from build123d import *

# Parameters (mm, degrees)
SKETCH_1_R          = 0.7
EXTRUDE_1_DEPTH     = 1
CUT_EXTRUDE_1_DEPTH = 2


with BuildPart() as part:
    # Эскиз1 → Вытянуть1 (new body)
    with BuildSketch(Plane(origin=(0, 0, 0), x_dir=(0, 0, -1), z_dir=(1, 0, 0))):
        with BuildLine():
            Line((0, 0), (70, 0))
            ThreePointArc((70, 0), (72, -2), (70, -4))
            Line((70, -4), (0, -4))
            ThreePointArc((0, -4), (-2, -2), (0, 0))
        make_face()
        with Locations((0, -2)):
            Circle(SKETCH_1_R, mode=Mode.SUBTRACT)
        with Locations((70, -2)):
            Circle(SKETCH_1_R, mode=Mode.SUBTRACT)
    extrude(amount=EXTRUDE_1_DEPTH)

    # Эскиз2 → Вырез-Вытянуть1 (cut, through all)
    with BuildSketch(Plane(origin=(1, 0, 0), x_dir=(0, 0, -1), z_dir=(1, 0, 0))):
        with BuildLine():
            Line((185.588178167, -105.966859724), (69.968626967, -4))
            ThreePointArc((69.968626967, -4), (67.624087686, -2.723985874), (64.958110934, -2.591153482))
            Line((64.958110934, -2.591153482), (56.968145289, -4))
            Line((56.968145289, -4), (-94.849228607, -30.769499158))
            Line((-94.849228607, -30.769499158), (-174.701887648, -328.568151357))
            Line((-174.701887648, -328.568151357), (105.735519126, -403.765511923))
            Line((105.735519126, -403.765511923), (185.588178167, -105.966859724))
        make_face()
    extrude(amount=-CUT_EXTRUDE_1_DEPTH, mode=Mode.SUBTRACT)


solid = part.part
Model file for the job. Use its own axes, mm. Coordinates: 2 decimals unless noted, no trailing zeros. Write each loop counter-clockwise with the first axis right and the second up, starting at its lowest first coordinate (ties: lowest second). Pieces come first, ordered by that corner, then holes. Notation, with made-up numbers: (60, -33.75) -> (111, -33.75) arc R25 ccw to (111, -14.75) -> close; hole circle Ø8 at (-36.75, 55). An arc over 180 degrees is marked (long way). One line per item, written item: value. Start each with the question number.
1) Slice it at A-A on x = 0.7. Count the separate pieces of the cut face and the enclosed holes in it, then the cut area to 3 significant figures.
2) Slice it at B-B on z = -61. Write the cut outline in (x, y), then the cut area to 3 significant figures.
3) Probe probe 1 along Y at (x, z) = (0.6, -70); probe 2 along Y at (x, z) = (0.5, -57); probe 3 along Y at (x, z) = (0.7, -68.5). List the from-to ranges inside material, lowest first.
4) Flat gauge pins, fed straight in: pin 1 Ø2 at (y, z) = (-2, 0) entering from +X; pin 2 Ø1.1 at (y, z) = (-2, -70) entering from +X. Where does each tip first touch, or does it go through?
5) Pull direction Z, two halves, no side cores. Call faces 1 (the face through (0.5, -2, -69.3)), 2 (the face through (0, -2, -36)), 3 (the face through (0.5, -2, -72)), 4 (the face through (0.507, -3.286, -61.019)): +Z half, -Z half, draft (parallel to the pull), parting line (faces both ways), or undercut.
Answers follow:
1. separate pieces: 1
1. enclosed holes: 2
1. area: 278 mm2
2. outline: (0, -3.29) -> (1, -3.29) -> (1, 0) -> (0, 0) -> close
2. area: 3.29 mm2
3. probe 1: -4 to -2.7, -1.3 to 0
3. probe 2: -3.99 to 0
3. probe 3: -3.05 to 0
4. pin 1: x = 1
4. pin 2: through
5. face 1: undercut
5. face 2: draft
5. face 3: -Z half
5. face 4: undercut
